Part model, mm, in its own coordinate system. Face numbers are marked on the shaded views. A direction names the side the tool comes from. Coordinates: 2 decimals unless noted, no trailing zeros. Order: outer loops, then holes, each group sorted by start corner. A loop starts at its lowest first (then second) coordinate and runs counter-clockwise, first axis right, second up.
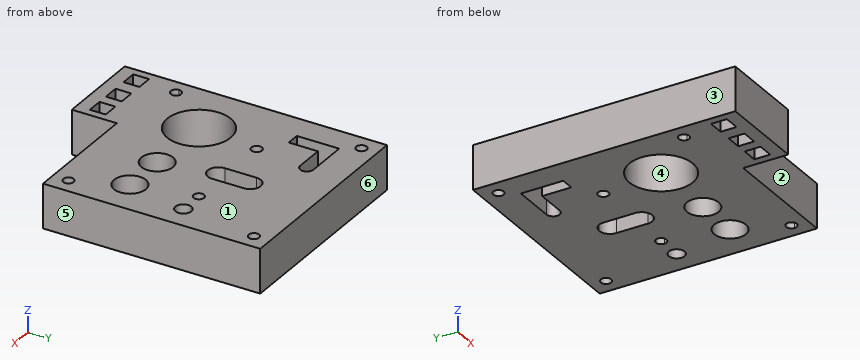
from build123d import *

# Parameters (mm, degrees)
F0_W     = 9
F0_H     = 9
F0_R     = 18
F0_R_2   = 9
F0_R_3   = 3
F0_R_4   = 4.5
F1_DEPTH = 25


with BuildPart() as f1:
    # F0 (on Top) → F1 (new body)
    with BuildSketch(Plane.XY):
        with BuildLine():
            Line((9, 0), (0, 0))
            Line((0, 0), (0, -9))
            Line((0, -9), (0, -18))
            Line((0, -18), (0, -52))
            Line((0, -52), (0, -114))
            Line((0, -114), (0, -132))
            Line((0, -132), (0, -148.5))
            Line((0, -148.5), (49.5, -148.5))
            Line((49.5, -148.5), (49.5, -123))
            Line((49.5, -123), (109.5, -123))
            Line((109.5, -123), (109.5, -117))
            ThreePointArc((109.5, -117), (107.3786796564, -111.8786796564), (112.5, -114))
            Line((112.5, -114), (118.5, -114))
            Line((118.5, -114), (118.5, -86.5))
            Line((118.5, -86.5), (118.5, -9))
            Line((118.5, -9), (118.5, 0))
            Line((118.5, 0), (109.5, 0))
            Line((109.5, 0), (90, 0))
            Line((90, 0), (66, 0))
            Line((66, 0), (39, 0))
            Line((39, 0), (9, 0))
        make_face()
        with Locations((9, -136.5)):
            Rectangle(F0_W, F0_H, mode=Mode.SUBTRACT)
        with Locations((25.5, -136.5)):
            Rectangle(F0_W, F0_H, mode=Mode.SUBTRACT)
        with BuildLine():
            ThreePointArc((9, -117), (6.8786796564, -116.1213203436), (6, -114))
            ThreePointArc((6, -114), (9, -111), (12, -114))
            ThreePointArc((12, -114), (11.1213203436, -116.1213203436), (9, -117))
        make_face(mode=Mode.SUBTRACT)
        with Locations((40.5, -136.5)):
            Rectangle(F0_W, F0_H, mode=Mode.SUBTRACT)
        with Locations((33, -86.5)):
            Circle(F0_R, mode=Mode.SUBTRACT)
        with Locations((72, -86.5)):
            Circle(F0_R_2, mode=Mode.SUBTRACT)
        with Locations((97.5, -86.5)):
            Circle(F0_R_2, mode=Mode.SUBTRACT)
        with BuildLine():
            ThreePointArc((39, -52), (36, -55), (33, -52))
            ThreePointArc((33, -52), (36, -49), (39, -52))
        make_face(mode=Mode.SUBTRACT)
        with BuildLine():
            Line((15, -18), (39, -18))
            ThreePointArc((39, -18), (42.75, -21.75), (39, -25.5))
            Line((39, -25.5), (22.5, -25.5))
            Line((22.5, -25.5), (22.5, -42))
            Line((22.5, -42), (15, -42))
            Line((15, -42), (15, -18))
        make_face(mode=Mode.SUBTRACT)
        with Locations((9, -9)):
            Circle(F0_R_3, mode=Mode.SUBTRACT)
        with BuildLine():
            ThreePointArc((66, -31.5), (70.2426406871, -33.2573593129), (72, -37.5))
            Line((72, -37.5), (72, -55.5))
            ThreePointArc((72, -55.5), (66, -61.5), (60, -55.5))
            Line((60, -55.5), (60, -37.5))
            ThreePointArc((60, -37.5), (61.7573593129, -33.2573593129), (66, -31.5))
        make_face(mode=Mode.SUBTRACT)
        with BuildLine():
            ThreePointArc((90, -49), (92.1213203436, -49.8786796564), (93, -52))
            ThreePointArc((93, -52), (87.8786796564, -54.1213203436), (90, -49))
        make_face(mode=Mode.SUBTRACT)
        with Locations((104.5, -52)):
            Circle(F0_R_4, mode=Mode.SUBTRACT)
        with Locations((109.5, -9)):
            Circle(F0_R_3, mode=Mode.SUBTRACT)
        with BuildLine():
            Line((118.5, -123), (118.5, -114))
            Line((118.5, -114), (112.5, -114))
            ThreePointArc((112.5, -114), (111.6213203436, -116.1213203436), (109.5, -117))
            Line((109.5, -117), (109.5, -123))
            Line((109.5, -123), (118.5, -123))
        make_face()
    extrude(amount=F1_DEPTH)


solid = f1.part
Q1. Cut at B-B on z = 18.75. Count the separate pieces of the cut face and the enclosed holes in it, and give its area (3 significant figures).
Results list:
separate pieces: 1
enclosed holes: 15
area: 13,200 mm2
Q2. Which spindle directions (+Z, -Z, +X, -X, +Y, -Y) get a long thin tool onto all of the face, cutting with end or side? Do the marked faces 1 and 2. Say none if no direction does.
Results list:
face 1: +Z, +X, -X, +Y, -Y
face 2: +Z, -Z, +X, -Y
Q3. Pin check, flat tips, straight feed: pin 1 Ø1 at (x, z) = (84.5, 17.5) entering from -Y; pin 2 Ø4.5 at (y, z) = (-138, 16.5) entering from +X. Stop position of each tip, or through.
Results list:
pin 1: stops at y = -123
pin 2: stops at x = 49.5
Q4. Cut at A-A on x = 97.5. Write the cut outline in (y, z).
Results list:
outline: (-123, 0) - (-95.5, 0) - (-95.5, 25) - (-123, 25) - close; (-77.5, 0) - (0, 0) - (0, 25) - (-77.5, 25) - close
Q5. Cut at C-C on x = 79. Write the cut outline in (y, z).
Results list:
outline: (-123, 0) - (-92.16, 0) - (-92.16, 25) - (-123, 25) - close; (-80.84, 0) - (0, 0) - (0, 25) - (-80.84, 25) - close
Q6. Wall check: line 1 along X through (y, z) = (-86, 13); line 2 along X through (y, z) = (-135.5, 9); line 3 along X through (y, z) = (-114, 8.25). Give the ranges that are in metal, low to high.
Results list:
line 1: x = 0 to 15.01, 50.99 to 63.01, 80.99 to 88.51, 106.49 to 118.5
line 2: x = 0 to 4.5, 13.5 to 21, 30 to 36, 45 to 49.5
line 3: x = 0 to 6, 12 to 106.5, 112.5 to 118.5
Q7. Mould opens along X. For the marked faces 3, 4, 5 and 6 say: pulls with the +X half, pulls with the -X half, needs draft (parallel to the pull), parting line crosses it, or undercut.
Results list:
face 3: pulls with the -X half
face 4: undercut
face 5: pulls with the +X half
face 6: needs draft
